Can you work these out from the model? Positions are in its coordinate system, mm. Give positions to 0.01 mm unless a question says otherwise; leave off trailing zeros. Order: outer loops, then holes, each group sorted by start corner. A loop starts at its lowest first (then second) coordinate and runs counter-clockwise, first axis right, second up.
Item 1: If I drill on line 1 along X through (y, z) = (3.75, 0.2); line 2 along X through (y, z) = (-0.75, -1.1); line 3 along Y through (x, z) = (2.25, -1.1), over which ranges is the centre line in solid material (lowest first)?
Item 2: If we mould it in two halves opening along Z, with no side actions, what happens to faces 1 (the flat face through (0, 0.572, -1)), 2 (the flat face through (0, 0, 1.245)), 3 (the flat face through (0, -0.572, 1)), 4 (the flat face through (3, 0, -1.245))? For each: +Z half, -Z half, draft (parallel to the pull), parting line (faces both ways), or undercut.
Item 3: I want a section at C-C, the plane z = 1. Count the separate pieces of the cut face and the enclosed holes in it, then the cut area to 3 significant figures.
Item 4: I want a section at B-B, the plane x = 3. Write out the boundary of the cut face in (y, z), then the cut area to 3 significant figures.
Item 5: I'm going to push flat-ended pins straight in: pin 1 Ø4 at (x, y) = (0.5, 3) entering from -Z; pin 2 Ø0.5 at (x, y) = (-2.5, 3.5) entering from +Z; pin 3 Ø0.7 at (y, z) = (2.5, 0) entering from +X. Where does each tip first touch, or does it pass through?
Item 6: I want a section at D-D, the plane z = 0.45. Write out the boundary of the cut face in (x, y).
Item 7: I want a section at A-A, the plane y = 1. Write out the boundary of the cut face in (x, z).
```python
from build123d import *

# Parameters (mm, degrees)
SKETCH1_W                        = 7.62
SKETCH1_H                        = 2.4892
BASE_EXTRUDE_DEPTH               = 0.5715
SNAP_GROOVES_DEPTH               = 2.143
SKETCH4_W                        = 0.4318
SKETCH4_H                        = 0.4318
STANDOFFS_DEPTH                  = 0.381
POSITION_PATTERN_COUNT           = 3
POSITION_PATTERN_PITCH           = 2.54
SKETCH5_W                        = 0.635
SKETCH5_H                        = 10
TERMINAL_TH_DEPTH                = 0.3175
T1_TIP1_SIZE                     = 0.2286
TERMINAL_PATTERN_COUNT           = 3
TERMINAL_PATTERN_PITCH           = 2.54
T1_TIP1_OF_TERMINAL_PATTERN_SIZE = 0.2286


with BuildPart() as part:
    # Sketch1 → Base-Extrude (new body, symmetric)
    with BuildSketch(Plane(origin=(0, 0, 0), x_dir=(1, 0, 0), z_dir=(0, 1, 0))):
        Rectangle(SKETCH1_W, SKETCH1_H)
    extrude(amount=BASE_EXTRUDE_DEPTH, both=True)

    # Sketch3 → Snap Grooves (cut, through all)
    with BuildSketch(Plane(origin=(0, 0.5715, 0), x_dir=(-1, 0, 0), z_dir=(0, 1, 0))):
        Polygon((1.016, 1.2446), (1.524, 1.2446), (1.27, 0.7366), align=None)
        Polygon((1.016, -1.2446), (1.524, -1.2446), (1.27, -0.7366), align=None)
        Polygon((3.81, -0.7366), (4.064, -1.2446), (3.556, -1.2446), align=None)
        Polygon((3.81, 0.7366), (4.064, 1.2446), (3.556, 1.2446), align=None)
    snap_grooves = extrude(amount=-SNAP_GROOVES_DEPTH, mode=Mode.SUBTRACT)

    # Sketch4 → Standoffs (add)
    with BuildSketch(Plane.XZ.offset(0.5715)):
        with Locations((-3.3401, 1.0287)):
            Rectangle(SKETCH4_W, SKETCH4_H)
        with Locations((-1.7399, 1.0287)):
            Rectangle(SKETCH4_W, SKETCH4_H)
        with Locations((-1.7399, -1.0287)):
            Rectangle(SKETCH4_W, SKETCH4_H)
        with Locations((-3.3401, -1.0287)):
            Rectangle(SKETCH4_W, SKETCH4_H)
    standoffs = extrude(amount=STANDOFFS_DEPTH)

    # Position Pattern: Snap Grooves, Standoffs ×3
    with Locations(*[(i * POSITION_PATTERN_PITCH, 0, 0) for i in range(1, POSITION_PATTERN_COUNT)]):
        add(snap_grooves, mode=Mode.SUBTRACT)
        add(standoffs)

    # Sketch5 → Terminal -TH (add, symmetric)
    with BuildSketch(Plane.ZY.offset(2.54)):
        with Locations((0, 1.4135)):
            Rectangle(SKETCH5_W, SKETCH5_H)
    terminal_th = extrude(amount=TERMINAL_TH_DEPTH, both=True)

    # T1 Tip1
    t1_tip1_edges = [part.edges().sort_by_distance(p)[0] for p in [
        (-2.54, -3.5865, 0.3175),
        (-2.8575, -3.5865, 0),
        (-2.54, 6.4135, -0.3175),
        (-2.2225, -3.5865, 0),
        (-2.54, -3.5865, -0.3175),
        (-2.2225, 6.4135, 0),
        (-2.54, 6.4135, 0.3175),
        (-2.8575, 6.4135, 0),
    ]]
    chamfer(t1_tip1_edges, length=T1_TIP1_SIZE)

    # Terminal Pattern: Terminal -TH ×3
    with Locations(*[(i * TERMINAL_PATTERN_PITCH, 0, 0) for i in range(1, TERMINAL_PATTERN_COUNT)]):
        add(terminal_th)

    # T1 Tip1 of Terminal Pattern
    t1_tip1_of_terminal_pattern_edges = [part.edges().sort_by_distance(p)[0] for p in [
        (0, -3.5865, 0.3175),
        (-0.3175, -3.5865, 0),
        (0, 6.4135, -0.3175),
        (0.3175, -3.5865, 0),
        (0, -3.5865, -0.3175),
        (0.3175, 6.4135, 0),
        (0, 6.4135, 0.3175),
        (-0.3175, 6.4135, 0),
        (2.54, -3.5865, 0.3175),
        (2.2225, -3.5865, 0),
        (2.54, 6.4135, -0.3175),
        (2.8575, -3.5865, 0),
        (2.54, -3.5865, -0.3175),
        (2.8575, 6.4135, 0),
        (2.54, 6.4135, 0.3175),
        (2.2225, 6.4135, 0),
    ]]
    chamfer(t1_tip1_of_terminal_pattern_edges, length=T1_TIP1_OF_TERMINAL_PATTERN_SIZE)


solid = part.part
```
Results list:
1. line 1: x = -2.86 to -2.22, -0.32 to 0.32, 2.22 to 2.86
1. line 2: x = -3.56 to -3.12, -1.96 to -1.52, -1.02 to -0.58, 0.58 to 1.02, 1.52 to 1.96, 3.12 to 3.56
1. line 3: y = -0.57 to 0.57
2. face 1: draft
2. face 2: +Z half
2. face 3: undercut
2. face 4: -Z half
3. separate pieces: 3
3. enclosed holes: 0
3. area: 8.79 mm2
4. outline: (-0.57, -1.24) - (0.57, -1.24) - (0.57, 1.24) - (-0.57, 1.24) - close
4. area: 2.85 mm2
5. pin 1: stops at z = -0.32
5. pin 2: stops at z = 0.32
5. pin 3: stops at x = 2.86
6. outline: (-3.81, -0.57) - (3.81, -0.57) - (3.81, 0.57) - (-3.81, 0.57) - close
7. outline: (-2.86, -0.32) - (-2.22, -0.32) - (-2.22, 0.32) - (-2.86, 0.32) - close; (-0.32, -0.32) - (0.32, -0.32) - (0.32, 0.32) - (-0.32, 0.32) - close; (2.22, -0.32) - (2.86, -0.32) - (2.86, 0.32) - (2.22, 0.32) - close
